Autodesk Inventor part; units mm, degrees
ref_plane "YZ Plane" through (0, 0, 0) normal (1, 0, 0) x (0, 1, 0)
ref_plane "XZ Plane" through (0, 0, 0) normal (0, 1, 0) x (-1, 0, 0)
ref_plane "XY Plane" through (0, 0, 0) normal (0, 0, 1) x (1, 0, 0)
sketch "Sketch1" plane through (0, 0, 0) normal (0, 1, 0) x (-1, 0, 0)
  line L0 (0, 0) -> (75, 0)
  line L1 (75, 0) -> (75, -98)
  line L2 (75, -98) -> (0, -98)
  line L3 (0, -98) -> (0, 0)
  dimension "d0" = 75
  dimension "d1" = 98
extrude "Extrusion1" add sketch "Sketch1" along normal blind 2
sketch "Sketch2" plane through (0, 2, 0) normal (0, 1, 0) x (1, 0, 0)
  line L0 (-75, 0) -> (0, 0)
  line L1 (0, 0) -> (0, 98)
  line L2 (0, 98) -> (-75, 98)
  line L3 (-75, 98) -> (-75, 0)
  line L4 (-73, 2) -> (-2, 2)
  line L5 (-2, 2) -> (-2, 96)
  line L6 (-2, 96) -> (-73, 96)
  line L7 (-73, 96) -> (-73, 2)
  line L8 (-37.5, 2) -> (-37.5, 96)
  line L9 (-37.5, 0) -> (-37.5, 98)
  line L10 (-75, 0) -> (0, 0)
  line L11 (-37.5, 0) -> (-37.5, 98)
  line L12 (0, 98) -> (-75, 98)
  point P0 (-37.5, 49)
  dimension "d4" = 75
  dimension "d5" = 98
  dimension "d6" = 71
  dimension "d7" = 94
extrude "Extrusion2" add sketch "Sketch2" along normal blind 8 contours L3 L2 L9 L6 L7 L4 L0 | L9 L4 L5 L6 L2 L1 L0
sketch "Sketch5" plane through (0, 2, 0) normal (0, 1, 0) x (1, 0, 0)
  line L0 (-2, 2) -> (-73, 2)
  line L1 (-73, 96) -> (-2, 96)
  line L2 (-2, 2) -> (-73, 2)
  line L3 (-73, 2) -> (-73, 96)
  line L4 (-73, 96) -> (-2, 96)
  line L5 (-2, 96) -> (-2, 2)
  line L6 (-4, 4) -> (-71, 4)
  line L7 (-71, 4) -> (-71, 94)
  line L8 (-71, 94) -> (-4, 94)
  line L9 (-4, 94) -> (-4, 4)
  line L10 (-37.5, 4) -> (-37.5, 94)
  line L11 (-37.5, 2) -> (-37.5, 96)
  point P0 (0, 0)
  point P1 (-37.5, 49)
  dimension "d11" = 67
  dimension "d12" = 90
extrude "Extrusion3" add sketch "Sketch5" along normal blind 16 contours L0 L11 L6 L9 L8 L1 L5 | L0 L3 L1 L11 L8 L7 L6
fillet "Fillet2" radius 15 12 edges at (0, 5, 0) (-2, 14, -2) (0, 5, -98) (-2, 14, -96) (-75, 5, -98) (-73, 14, -96) (-71, 10, -4) (-75, 5, 0) (-73, 14, -2) (-4, 10, -4) (-71, 10, -94) (-4, 10, -94)
sketch "Sketch6" plane through (0, 2, 0) normal (0, 1, 0) x (1, 0, 0)
  line L0 (-18.5, 14) -> (-56.5, 14)
  line L1 (-56.5, 14) -> (-56.5, 68)
  line L2 (-56.5, 68) -> (-18.5, 68)
  line L3 (-18.5, 68) -> (-18.5, 14)
  line L4 (-18.5, 14) -> (-33.5, 14)
  line L5 (-33.5, 14) -> (-33.5, 16.5)
  line L6 (-33.5, 16.5) -> (-18.5, 16.5)
  line L7 (-18.5, 16.5) -> (-18.5, 14)
  line L8 (-18.5, 14) -> (-27, 14)
  line L9 (-27, 14) -> (-27, 55)
  line L10 (-27, 55) -> (-18.5, 55)
  line L11 (-18.5, 55) -> (-18.5, 14)
  circle A0 centre (-33.5, 16.5) radius 3
  circle A1 centre (-27, 55) radius 3
  line L12 (-19, 4) -> (-56, 4)
  line L13 (-37.5, 4) -> (-37.5, 94)
  line L14 (-19, 94) -> (-56, 94)
  line L15 (-37.5, 4) -> (-39.5, 4)
  line L16 (-39.5, 4) -> (-39.5, 14)
  line L17 (-39.5, 14) -> (-37.5, 14)
  line L18 (-37.5, 14) -> (-37.5, 4)
  point P0 (0, 0)
  dimension "d16" = 38
  dimension "d17" = 54
  dimension "d18" = 15
  dimension "d19" = 2.5
  dimension "d20" = 8.5
  dimension "d21" = 41
  dimension "d22" = 6
  dimension "d23" = 6
  dimension "d24" = 2
  dimension "d25" = 10
extrude "Extrusion4" add sketch "Sketch6" along normal blind 2 contours A0 L0 | L0 L5 L6 A0 | L0 A0 L6 L5 | A1 L10 L9 | L9 L10 A1
sketch "Sketch7" plane through (-33.5, 4, -16.5) normal (0, 1, 0) x (1, 0, 0)
  circle A0 centre (0, 0) radius 3
  circle A1 centre (0, 0) radius 1.5
  circle A2 centre (6.5, 38.5) radius 3
  circle A3 centre (6.5, 38.5) radius 1.5
  point P0 (33.5, -16.5)
  dimension "d28" = 3
  dimension "d29" = 3
extrude "Extrusion5" cut sketch "Sketch7" against normal blind 3 contours A1 | A3
sketch "Sketch8" plane through (-17, 18, -96) normal (0, 0, -1) x (-1, 0, 0)
  line L0 (41, -8) -> (41, 0)
  line L1 (41, -8) -> (0, -8)
  line L2 (0, -8) -> (0, -3)
  line L3 (0, -3) -> (41, -3)
  line L4 (41, -3) -> (41, -8)
  circle A0 centre (20.5, -3) radius 1.5
  point P0 (-17, -18)
  dimension "d32" = 41
  dimension "d33" = 5
  dimension "d34" = 3
extrude "Extrusion6" cut sketch "Sketch8" against normal blind 100 contours A0 L3 | L3 A0
sketch "Sketch9" plane through (0, 2, 0) normal (0, 1, 0) x (1, 0, 0)
  point P0 (0, 0)
sketch "Sketch10" plane through (-2, 10, -81) normal (1, 0, 0) x (0, 0, -1)
  line L0 (-66, -10) -> (-66, 0)
  line L1 (-66, 0) -> (-46, 0)
  line L2 (-46, 0) -> (-46, 2.5)
  line L3 (-46, 2.5) -> (-66, 2.5)
  line L4 (-66, 2.5) -> (-66, 0)
  line L5 (-66, 0) -> (-36, 0)
  line L6 (-36, 0) -> (-36, 2.5)
  line L7 (-36, 2.5) -> (-66, 2.5)
  line L8 (-66, 2.5) -> (-66, 0)
  circle A0 centre (-46, 2.5) radius 2.5
  circle A1 centre (-36, 2.5) radius 2.5
  line L9 (-48.5, 2.5) -> (-48.5, 8)
  line L10 (-2, 8) -> (-62, 8)
  line L11 (-43.5, 2.5) -> (-43.5, 8)
  line L12 (-38.5, 2.5) -> (-38.5, 8)
  line L13 (-33.5, 2.5) -> (-33.5, 8)
  point P0 (-81, -10)
  dimension "d37" = 20
  dimension "d38" = 2.5
  dimension "d39" = 30
  dimension "d40" = 2.5
  dimension "d41" = 5
  dimension "d42" = 5
extrude "Extrusion7" cut sketch "Sketch10" against normal blind 5 contours A0 L3 L2 | L2 L7 A0 | L3 A0 L7 | A1 L7 L6 | L6 L7 A1 | L9 L10 L11 A0 | L12 L10 L13 A1
properties part number "reduced_tortoise_3_base"
Input: part model. Units: mm. Frame: model coordinates. A direction names the side the tool comes from. Round coordinates to 2 decimals unless told otherwise and drop trailing zeros. Loops run counter-clockwise (first coordinate to the right, second up) from the corner with the lowest first, then second, coordinate; pieces in that order, holes last. Notation, with made-up numbers: (27.5, 20.5) -> (38.5, 20.5) arc R22 cw to (38.5, 52.5) -> close; hole circle Ø10 at (76, 60). An arc over 180 degrees is marked (long way). Use one line per item in the form item = value. Start each with the question number.
Item 1: Mould query, pull axis X, two halves, no side actions, for faces 5 (the face through (-2, 14, -24)), 6 (the face through (-75, 5, -49)), 7 (the face through (-8.28, 10.11, -89.49)). Classes: pulls with the +X half, pulls with the -X half, needs draft (parallel to the pull), parting line crosses it, or undercut.
Item 2: Section query B-B on x = -37.5. Return the cut outline in (y, z).
Item 3: Section query A-A on y = 15. Count the separate pieces of the cut face and the enclosed holes in it, then the cut area to 3 significant figures.
Item 4: Section query C-C on y = 5. Return the cut outline in (x, z).
Item 5: Section query D-D on x = -27. Return the cut outline in (y, z).
Item 6: Contact query for flat-ended pins moving along their axis: pin 1 Ø0.9 at (x, z) = (-27, -55) entering from +Y; pin 2 Ø6.5 at (y, z) = (15.5, -42) entering from +X; pin 3 Ø3 at (x, z) = (-55, -21.5) entering from +Y. Output: stop coordinate, or through.
Item 7: Material intervals for L1, parallel to Z at x = -33.5, y = 3.25; L2, parallel to Z at x = -39.5, y = 11.75; L3, parallel to X at y = 11, z = -63, sorted ascending. Write a range as from..to.
Item 8: Set-up query: faces 1 (the face through (-38, 13, -96)), 2 (the face through (-3, 15, -32.5)), 3 (the face through (-27, 3, -52)), 4 (the face through (-68.49, 14.06, -91.72)). Return all of +Z, -Z, +X, -X, +Y, -Y with unobstructed straight access to the full face (end or side cutting, diameter ignored); none if empty.
Ans:
q1.face_5 = pulls with the +X half
q1.face_6 = pulls with the -X half
q1.face_7 = undercut
q2.outline = (0, -98) -> (10, -98) -> (10, -96) -> (13.5, -96) -> (13.5, -94) -> (2, -94) -> (2, -4) -> (13.5, -4) -> (13.5, -2) -> (10, -2) -> (10, 0) -> (0, 0) -> close; (16.5, -96) -> (18, -96) -> (18, -94) -> (16.5, -94) -> close; (16.5, -4) -> (18, -4) -> (18, -2) -> (16.5, -2) -> close
q3.separate_pieces = 4
q3.enclosed_holes = 0
q3.area = 612 mm^2
q4.outline = (-75, -83) arc R15 ccw to (-60, -98) -> (-15, -98) arc R15 ccw to (0, -83) -> (0, -15) arc R15 ccw to (-15, 0) -> (-60, 0) arc R15 ccw to (-75, -15) -> close; hole (-71, -79) arc R15 ccw to (-56, -94) -> (-19, -94) arc R15 ccw to (-4, -79) -> (-4, -19) arc R15 ccw to (-19, -4) -> (-56, -4) arc R15 ccw to (-71, -19) -> close
q5.outline = (0, -98) -> (10, -98) -> (10, -96) -> (18, -96) -> (18, -94) -> (2, -94) -> (2, -58) -> (4, -58) -> (4, -56.5) -> (1, -56.5) -> (1, -53.5) -> (4, -53.5) -> (4, -52) -> (2, -52) -> (2, -4) -> (18, -4) -> (18, -2) -> (10, -2) -> (10, 0) -> (0, 0) -> close
q6.pin_1 = 1
q6.pin_2 = -2
q6.pin_3 = 2
q7.L1 = -98..-94, -19.5..-18, -15..-13.5, -4..0
q7.L2 = -96..-94, -4..-2
q7.L3 = -73..-71, -4..-2
q8.face_1 = -Z, +X, -X, +Y
q8.face_2 = +X, +Y
q8.face_3 = +Y
q8.face_4 = -Z, -X, +Y
